```python
from build123d import *

# Parameters (mm, degrees)
SKETCH_R           = 18
PAD_DEPTH          = 10
SKETCH001_R        = 22
POCKET_DEPTH       = 8.4
SKETCH002_R        = 6.4
POCKET001_DEPTH    = 17
SKETCH003_R        = 5
POCKET002_DEPTH    = 5
SKETCH004_R        = 1
POCKET003_DEPTH    = 8
POLARPATTERN_COUNT = 5
POCKET004_DEPTH    = 3
SKETCH006_R        = 2
POCKET005_DEPTH    = 5
FILLET_R           = 4
FILLET001_R        = 1


with BuildPart() as part:
    # Sketch → Pad (new body)
    with BuildSketch(Plane.XY):
        with BuildLine():
            Line((-8, -40), (8, -40))
            Line((8, -40), (8, -26.832816))
            ThreePointArc((8, -26.832816), (0, 28), (-8, -26.832816))
            Line((-8, -26.832816), (-8, -40))
        make_face()
        Circle(SKETCH_R, mode=Mode.SUBTRACT)
    extrude(amount=PAD_DEPTH)

    # Sketch001 (on Face6 of Pad) → Pocket (cut)
    with BuildSketch(Plane(origin=(0, 0, 0), x_dir=(1, 0, 0), z_dir=(0, 0, -1))):
        Circle(SKETCH001_R)
    extrude(amount=-POCKET_DEPTH, mode=Mode.SUBTRACT)

    # Sketch002 (on Face1 of Pocket) → Pocket001 (cut)
    with BuildSketch(Plane.XZ.offset(40)):
        Circle(SKETCH002_R)
    extrude(amount=-POCKET001_DEPTH, mode=Mode.SUBTRACT)

    # Sketch003 (on Face7 of Pocket001) → Pocket002 (cut)
    with BuildSketch(Plane.XZ.offset(23)):
        Circle(SKETCH003_R)
    extrude(amount=-POCKET002_DEPTH, mode=Mode.SUBTRACT)

    # Sketch004 (on Face2 of Pocket002) → Pocket003 (cut)
    with BuildSketch(Plane(origin=(0, 0, 0), x_dir=(1, 0, 0), z_dir=(0, 0, -1))):
        with Locations((0, -25)):
            Circle(SKETCH004_R)
    pocket003 = extrude(amount=-POCKET003_DEPTH, mode=Mode.SUBTRACT)

    # PolarPattern: Pocket003 ×5 about axis
    polarpattern_axis = Axis((0, 0, 0), (0, 0, -1))
    for i in range(1, POLARPATTERN_COUNT):
        add(pocket003.rotate(polarpattern_axis, i * 360 / POLARPATTERN_COUNT), mode=Mode.SUBTRACT)

    # Sketch005 → Pocket004 (cut)
    with BuildSketch(Plane.XY.offset(10)):
        Polygon((0, -36.041452), (3.5, -34.020726), (3.5, -29.979274), (0, -27.958548), (-3.5, -29.979274), (-3.5, -34.020726), align=None)
    extrude(amount=-POCKET004_DEPTH, mode=Mode.SUBTRACT)

    # Sketch006 (on Face29 of Pocket004) → Pocket005 (cut)
    with BuildSketch(Plane.XY.offset(7)):
        with Locations((0, -32)):
            Circle(SKETCH006_R)
    extrude(amount=-POCKET005_DEPTH, mode=Mode.SUBTRACT)

    # Fillet
    fillet_edges = [part.edges().sort_by_distance(p)[0] for p in [
        (0, 28, 10),
        (8, -33.416408, 10),
        (-8, -33.416408, 10),
    ]]
    fillet(fillet_edges, radius=FILLET_R)

    # Fillet001
    fillet001_edges = [part.edges().sort_by_distance(p)[0] for p in [
        (-18, 0, 10),
    ]]
    fillet(fillet001_edges, radius=FILLET001_R)


solid = part.part
```
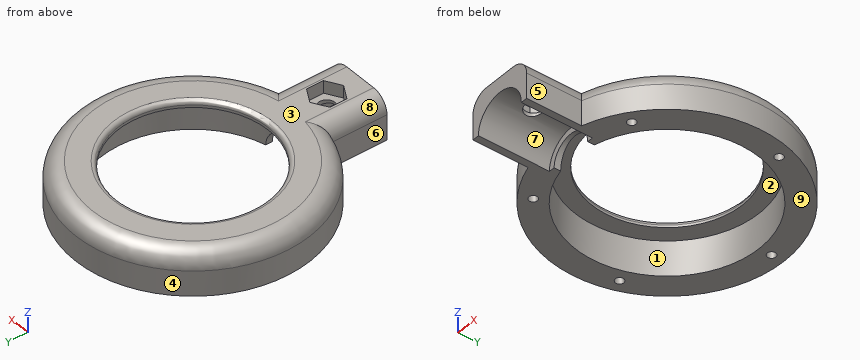
Source: CAD feature listing. Evaluate the final solid. Frame: model axes, mm. Face numbers are marked on the shaded views. A direction names the side the tool comes from. Round coordinates to 2 decimals unless told otherwise and drop trailing zeros. Loops run counter-clockwise (first coordinate to the right, second up) from the corner with the lowest first, then second, coordinate; pieces in that order, holes last. Notation, with made-up numbers: (11, 29.5) - (15, 29.5) arc R7 ccw to (15, 42.5) - close; hole circle Ø10 at (23, 56). An arc over 180 degrees is marked (long way). Use CSV: the item, a comma, the result in double quotes.
Q1. Reachability of the marked faces 5, 6, 7, 8 and 9 from +Z, -Z, +X, -X, +Y, -Y: full face, straight path, thin tool, end or side. Return the list, or none.
Reported:
face 5,"+Z, -Z, +X, -Y"
face 6,"+Z, -Z, -X, -Y"
face 7,"-Z, -Y"
face 8,"+Z, -X, -Y"
face 9,"-Z, +X, -X, +Y, -Y"
Q2. Mould query, pull axis Y, two halves, no side actions, for the marked faces 1, 2, 3 and 4. Classes: pulls with the +Y half, pulls with the -Y half, needs draft (parallel to the pull), parting line crosses it, or undercut.
Reported:
face 1,"undercut"
face 2,"undercut"
face 3,"needs draft"
face 4,"parting line crosses it"
Q3. Pin query (flat end, axial travel): pin 1 Ø1 at (x, y) = (-24, 7.5) entering from -Z; pin 2 Ø3 at (y, z) = (9.5, 5) entering from +X; pin 3 Ø1.5 at (y, z) = (-31, 8.5) entering from +X; pin 4 Ø10 at (x, y) = (0.5, -10.5) entering from +Z. Return the tip coordinate at first contact, or that it passes through.
Reported:
pin 1,"z = 8"
pin 2,"x = 26.83"
pin 3,"x = 7.6"
pin 4,"through"
Q4. Ray query, line 1 along X through (y, z) = (-36, 4); line 2 along Y through (x, z) = (0, 6.45); line 3 along Y through (x, z) = (-14.5, 1). Return the intervals inside material, ascending.
Reported:
line 1,"-8 to -5, 5 to 8"
line 2,"-40 to -34, -30 to -22, 22 to 24, 26 to 27.97"
line 3,"-23.95 to -21.21, -19.24 to -16.55, 16.55 to 23.95"
Q5. Section query B-B, the plane z = 3.75. Output: boundary loops of the cut face in (x, y).
Reported:
outline,"(-8, -40) - (-5.19, -40) - (-5.19, -23) - (-3.31, -23) - (-3.31, -21.75) arc R22 cw (long way) to (3.31, -21.75) - (3.31, -23) - (5.19, -23) - (5.19, -40) - (8, -40) - (8, -26.83) arc R28 ccw (long way) to (-8, -26.83) - close; hole circle Ø2 at (-23.78, 7.73); hole circle Ø2 at (-14.69, -20.23); hole circle Ø2 at (0, 25); hole circle Ø2 at (14.69, -20.23); hole circle Ø2 at (23.78, 7.73)"
Q6. Section query A-A, the plane y = -32. Output: boundary loops of the cut face in (x, z), then the cut area to 3 significant figures.
Reported:
outline,"(-8, 0) - (-6.4, 0) arc R6.4 cw to (-2, 6.08) - (-2, 7) - (-3.5, 7) - (-3.5, 10) - (-4, 10) arc R4 ccw to (-8, 6) - close; (2, 6.08) arc R6.4 cw to (6.4, 0) - (8, 0) - (8, 6) arc R4 ccw to (4, 10) - (3.5, 10) - (3.5, 7) - (2, 7) - close"
area,"65.0 mm^2"
